Work out the finished part from the listing and answer in its coordinate system (mm). Give positions to 0.01 mm unless a question says otherwise; leave off trailing zeros. Loops run counter-clockwise (first coordinate to the right, second up) from the corner with the lowest first, then second, coordinate; pieces in that order, holes last. Notation, with made-up numbers: (-9, 71) - (40, 71) arc R32 ccw to (40, 106) - close; hole circle Ø7 at (30, 75.25). An arc over 180 degrees is marked (long way). One line per question, with ' | ' between items. Start each with the question number.
1. Section D-D (y = 12.7) is taken. Determine the outline of the cut face in (x, z) (3 decimals).
2. Find the intervals of material crossed by line 1 (X direction, y = 158.75, z = 1.3); line 2 (X direction, y = 125, z = 2.9); line 3 (Y direction, x = 152, z = 1.4), in increasing order.
3. Section A-A (y = 97.79) is taken. Determine the outline of the cut face in (x, z) (1 decimal).
4. Section B-B (y = 46.99) is taken. Determine the outline of the cut face in (x, z) (3 decimals), plus the area to 3 significant figures.
5. Section C-C (z = 0.75) is taken. Give the number of separate pieces and of enclosed holes in the cut face, plus the area to 3 significant figures.
6. This flat-tipped pin is pushed along its axis until it touches: pin 1 (8.5 mm diameter, centred on x = 154.37, y = 124.78, fed in from +Z). Where does it stop, or does it pass through?
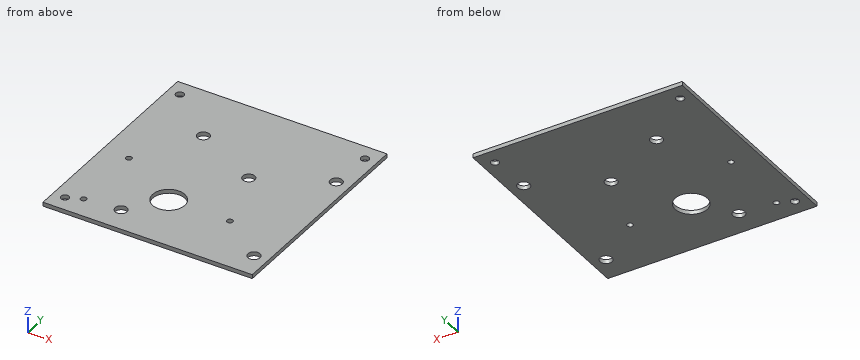
from build123d import *

# Parameters (mm, degrees)
SKETCH1_W           = 165.481
SKETCH1_H           = 171.45
SKETCH1_R           = 2.31775
SKETCH1_R_2         = 2.286
SKETCH1_R_3         = 12.7
SKETCH1_R_4         = 4.7625
BOSS_EXTRUDE1_DEPTH = 3.175
SKETCH2_R           = 3.175
CUT_EXTRUDE1_DEPTH  = 3.175


with BuildPart() as part:
    # Sketch1 → Boss-Extrude1 (new body)
    with BuildSketch(Plane.XY):
        with Locations((82.7405, 85.725)):
            Rectangle(SKETCH1_W, SKETCH1_H)
        with Locations((21.0185, 17.78)):
            Circle(SKETCH1_R, mode=Mode.SUBTRACT)
        with Locations((21.0185, 75.565)):
            Circle(SKETCH1_R_2, mode=Mode.SUBTRACT)
        with Locations((118.6307, 46.99)):
            Circle(SKETCH1_R, mode=Mode.SUBTRACT)
        with Locations((70.231, 46.99)):
            Circle(SKETCH1_R_3, mode=Mode.SUBTRACT)
        with Locations((101.981, 97.79)):
            Circle(SKETCH1_R_4, mode=Mode.SUBTRACT)
        with Locations((49.3395, 20.0025)):
            Circle(SKETCH1_R_4, mode=Mode.SUBTRACT)
        with Locations((49.3395, 124.7775)):
            Circle(SKETCH1_R_4, mode=Mode.SUBTRACT)
        with Locations((154.3685, 20.0025)):
            Circle(SKETCH1_R_4, mode=Mode.SUBTRACT)
        with Locations((154.3685, 124.7775)):
            Circle(SKETCH1_R_4, mode=Mode.SUBTRACT)
    extrude(amount=BOSS_EXTRUDE1_DEPTH)

    # Sketch2 → Cut-Extrude1 (cut)
    with BuildSketch(Plane.XY.offset(3.175)):
        with Locations((9.525, 158.75)):
            Circle(SKETCH2_R)
        with Locations((9.525, 12.7)):
            Circle(SKETCH2_R)
        with Locations((155.956, 158.75)):
            Circle(SKETCH2_R)
    extrude(amount=-CUT_EXTRUDE1_DEPTH, mode=Mode.SUBTRACT)


solid = part.part
Conclusion:
1) outline: (0, 0) - (6.35, 0) - (6.35, 3.175) - (0, 3.175) - close; (12.7, 0) - (165.481, 0) - (165.481, 3.175) - (12.7, 3.175) - close
2) line 1: 0 to 6.35, 12.7 to 152.78, 159.13 to 165.48 | line 2: 0 to 44.58, 54.1 to 149.61, 159.13 to 165.48 | line 3: 0 to 15.87, 24.13 to 120.65, 128.91 to 171.45
3) outline: (0, 0) - (97.2, 0) - (97.2, 3.2) - (0, 3.2) - close; (106.7, 0) - (165.5, 0) - (165.5, 3.2) - (106.7, 3.2) - close
4) outline: (0, 0) - (57.531, 0) - (57.531, 3.175) - (0, 3.175) - close; (82.931, 0) - (116.313, 0) - (116.313, 3.175) - (82.931, 3.175) - close; (120.948, 0) - (165.481, 0) - (165.481, 3.175) - (120.948, 3.175) - close | area: 430 mm²
5) separate pieces: 1 | enclosed holes: 12 | area: 27,400 mm²
6) pin 1: through
